Here's how the part is built. I have some questions about the finished solid (model axes, mm). Face numbers are marked on the shaded views. Coordinates: 2 decimals unless noted, no trailing zeros. Write each loop counter-clockwise with the first axis right and the second up, starting at its lowest first coordinate (ties: lowest second). Pieces come first, ordered by that corner, then holes.
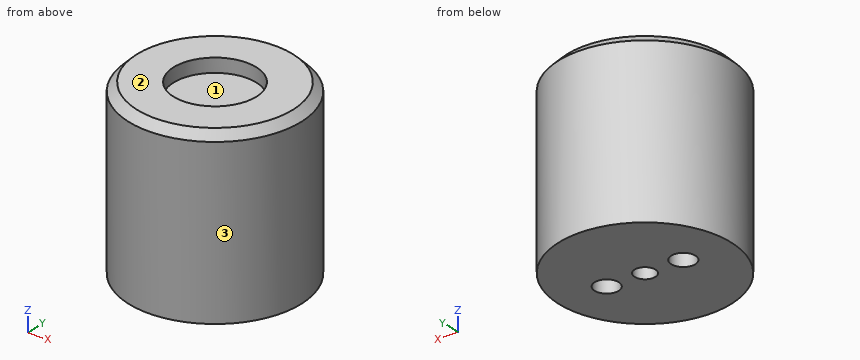
```python
from build123d import *

# Parameters (mm, degrees)
F0_R     = 12.5
F1_DEPTH = 25
F2_R     = 6
F3_DEPTH = 2
F5_DEPTH = 10
F6_SIZE  = 1.2


with BuildPart() as f1:
    # F0 (on Top) → F1 (new body)
    with BuildSketch(Plane.XY):
        Circle(F0_R)
    extrude(amount=F1_DEPTH)

    # F2 (on face) → F3 (cut)
    with BuildSketch(Plane.XY.offset(25)):
        Circle(F2_R)
    extrude(amount=-F3_DEPTH, mode=Mode.SUBTRACT)

    # F4 (on face) → F5 (cut)
    with BuildSketch(Plane(origin=(0, 0, 0), x_dir=(1, 0, 0), z_dir=(0, 0, -1))):
        with BuildLine():
            ThreePointArc((-3.75, 0), (-5.5, 1.75), (-7.25, 0))
            Line((-7.25, 0), (-3.75, 0))
        make_face()
        with BuildLine():
            ThreePointArc((7.25, 0), (5.5, 1.75), (3.75, 0))
            Line((3.75, 0), (7.25, 0))
        make_face()
        with BuildLine():
            Line((7.25, 0), (3.75, 0))
            ThreePointArc((3.75, 0), (5.5, -1.75), (7.25, 0))
        make_face()
        with BuildLine():
            ThreePointArc((1.5, 0), (0, 1.5), (-1.5, 0))
            Line((-1.5, 0), (1.5, 0))
        make_face()
        with BuildLine():
            Line((1.5, 0), (-1.5, 0))
            ThreePointArc((-1.5, 0), (0, -1.5), (1.5, 0))
        make_face()
        with BuildLine():
            Line((-3.75, 0), (-7.25, 0))
            ThreePointArc((-7.25, 0), (-5.5, -1.75), (-3.75, 0))
        make_face()
    extrude(amount=-F5_DEPTH, mode=Mode.SUBTRACT)

    # F6
    f6_edges = [f1.edges().sort_by_distance(p)[0] for p in [
        (-12.5, 0, 25),
    ]]
    chamfer(f6_edges, length=F6_SIZE)


solid = f1.part
```
1) We'd pull the mould along X, two halves only. Please class the marked faces 1, 2 and 3: pulls with the +X half, pulls with the -X half, needs draft (parallel to the pull), parting line crosses it, or undercut.
Values follow:
face 1: undercut
face 2: needs draft
face 3: parting line crosses it
2) I need wall thicknesses on probe 1 along Y at (x, z) = (0, 2.5); probe 2 along Y at (x, z) = (-4, 2.75); probe 3 along Y at (x, z) = (-6, 14.75). Which ranges of each line are inside material? Lowest first, please.
Values follow:
probe 1: y = -12.5 to -1.5, 1.5 to 12.5
probe 2: y = -11.84 to -0.9, 0.9 to 11.84
probe 3: y = -10.97 to 10.97
3) Imagine slicing it at C-C on z = 21.5. Please give me the cut outline in (x, y), then the cut area to 3 significant figures.
Values follow:
outline: circle Ø25 at (0, 0)
area: 491 mm2
4) Will these pins go through, and if not, where does the flat tip stop? pin 1 (2 mm diameter, centred on x = 8.5, z = 14.5, fed in from +Y); pin 2 (12 mm diameter, centred on y = -6.5, z = 14, fed in from -X); pin 3 (3.5 mm diameter, centred on x = 0, y = 2, fed in from +Z).
Values follow:
pin 1: stops at y = 10
pin 2: stops at x = -12.49
pin 3: stops at z = 23
5) Imagine slicing it at B-B on z = 8.75. Please give me the cut outline in (x, y), then the cut area to 3 significant figures.
Values follow:
outline: circle Ø25 at (0, 0); hole circle Ø3.5 at (-5.5, 0); hole circle Ø3 at (0, 0); hole circle Ø3.5 at (5.5, 0)
area: 465 mm2
6) Imagine slicing it at A-A on y = 0. Please give me the cut outline in (x, z).
Values follow:
outline: (-12.5, 0) - (-7.25, 0) - (-7.25, 10) - (-3.75, 10) - (-3.75, 0) - (-1.5, 0) - (-1.5, 10) - (1.5, 10) - (1.5, 0) - (3.75, 0) - (3.75, 10) - (7.25, 10) - (7.25, 0) - (12.5, 0) - (12.5, 23.8) - (11.3, 25) - (6, 25) - (6, 23) - (-6, 23) - (-6, 25) - (-11.3, 25) - (-12.5, 23.8) - close
